Autodesk Inventor part; units mm, degrees
ref_plane "YZ Plane" through (0, 0, 0) normal (1, 0, 0) x (0, 1, 0)
ref_plane "XZ Plane" through (0, 0, 0) normal (0, 1, 0) x (-1, 0, 0)
ref_plane "XY Plane" through (0, 0, 0) normal (0, 0, 1) x (1, 0, 0)
sketch "Sketch1" plane through (0, 0, 0) normal (1, 0, 0) x (0, 1, 0)
  circle A0 centre (0, 0) radius 3.175
  dimension "d0" = 6.35
extrude "Extrusion1" add sketch "Sketch1" along normal mid plane 63.5
sketch "Sketch2" plane through (0, 0, 0) normal (0, 1, 0) x (-1, 0, 0)
  circle A0 centre (-28.575, 0) radius 1.27
  line L0 (-31.75, 3.175) -> (-31.75, -3.175)
  point P0 (0, 0)
  dimension "d3" = 2.54
  dimension "d4" = 3.175
extrude "Extrusion2" cut sketch "Sketch2" along normal through all both and the other way through all
sketch "Sketch3" plane through (0, 0, 0) normal (0, 0, 1) x (1, 0, 0)
  circle A0 centre (40.64, 0) radius 12.7
  point P0 (0, 0)
  dimension "d7" = 25.4
  dimension "d8" = 40.64
sketch "Sketch4" plane through (0, 0, 0) normal (0, 1, 0) x (-1, 0, 0)
  line L0 (-27.94, 0) -> (-53.34, 0) construction
  circle A0 centre (-53.34, 0) radius 1.016
  point P0 (0, 0)
  dimension "d9" = 2.032
sweep "Sweep1" add profiles "Sketch4" path "Sketch3"
sketch "Sketch5" plane through (0, 0, 0) normal (0, 1, 0) x (-1, 0, 0)
  line L0 (28.575, 0) -> (28.575, -3.9688)
  arc A0 (26.9875, -2.3813) -> (28.575, -3.9688) centre (28.575, -2.3813) ccw
  line L1 (26.9875, -2.3813) -> (26.9875, 0)
  line L2 (26.9875, 0) -> (28.575, 0)
  line L3 (31.75, -3.175) -> (31.75, 3.175)
  point P0 (0, 0)
  dimension "d12" = 1.5875
  dimension "d13" = 3.175
  dimension "d14" = 0.7937
revolve "Revolution1" add sketch "Sketch5" angle 360 about axis through (-28.575, 0, 0) along (0, 0, -1)
chamfer "Chamfer1" distance 1.5875 angle 45 2 edges at (-31.75, -3.175, 0) (31.75, -3.175, 0)
properties part number "Release_Pin" material "Aluminum 6061"
Here's how the part is built. I have some questions about the finished solid (model axes, mm). Coordinates: 2 decimals unless noted, no trailing zeros. Order: outer loops, then holes, each group sorted by start corner. A loop starts at its lowest first (then second) coordinate and runs counter-clockwise, first axis right, second up.
1) Will these pins go through, and if not, where does the flat tip stop? pin 1 (12 mm diameter, centred on x = -11, y = 0.5, fed in from -Z) (3 decimals); pin 2 (1.5 mm diameter, centred on x = 5.5, y = -2.5, fed in from -Z); pin 3 (1.5 mm diameter, centred on x = 28.575, z = 0, fed in from +Y).
2) I need wall thicknesses on line 1 (X direction, y = -1.5, z = 0) (3 decimals); line 2 (X direction, y = 2, z = 0.5); line 3 (Y direction, x = 31.5, z = -1.5). Which ranges of each line are inside material? Lowest first, please.
3) Imagine slicing it at B-B on x = 11.5. List the corners of the cut face in (y, z) for me (3 decimals), and give its area (3 significant figures).
4) Imagine slicing it at A-A on y = 0. State how many separate pieces and enclosed holes the cut face has, and give its area (3 significant figures).
5) We'd pull the mould along Z, two halves only. Please class faces 1 (the face through (31.75, 0, 0)), 2 (the face through (29.844, -0.045, -0.051)), 3 (the face through (-0.42, -0.69, 3.1)): +Z half, -Z half, draft (parallel to the pull), parting line (faces both ways), or undercut.
Response values:
1. pin 1: stops at z = -3.175
1. pin 2: stops at z = -2.65
1. pin 3: stops at y = 7.75
2. line 1: x = -31.75 to 29.053, 29.845 to 31.75, 52.227 to 54.274
2. line 2: x = -31.28 to 28.99, 29.74 to 31.28, 52.29 to 54.08
2. line 3: y = -1.06 to 1.06
3. outline: circle Ø6.35 at (0, 0)
3. area: 31.7 mm2
4. separate pieces: 2
4. enclosed holes: 1
4. area: 401 mm2
5. face 1: draft
5. face 2: undercut
5. face 3: parting line
